Could you check a few things on this model? Use its own coordinates, in mm. Face numbers are marked on the shaded views. A direction names the side the tool comes from. Give positions to 0.01 mm unless a question says otherwise; leave off trailing zeros. Loops run counter-clockwise (first coordinate to the right, second up) from the corner with the lowest first, then second, coordinate; pieces in that order, holes last. Notation, with made-up numbers: (-27, 47) - (23, 47) arc R23 ccw to (23, 57) - close; hole circle Ø11 at (29.25, 44). An arc over 180 degrees is marked (long way). One line per item, written item: value. Start each with the question number.
Q1. I want a section at A-A (z = -18.5). Please give me the cut outline in (x, y), then the cut area to 3 significant figures.
Q2. I want a section at C-C (y = -44). Please give me the cut outline in (x, z), then the cut area to 3 significant figures.
Q3. I want a section at B-B (x = 0). Please give me the cut outline in (y, z), then the cut area to 3 significant figures.
Q4. For the marked faces 1, 2, 3, 4 and 5, which set-ups out of +Z, -Z, +X, -X, +Y, -Y let a thin tool reach every point of the face, with its end or its side?
Q5. I'm going to push flat-ended pins straight in: P1, Ø12, axis at y = -42.5, z = -20, coming from the -X side; P2, Ø2.5, axis at y = -17.5, z = -33, coming from the +X side; P3, Ø5.5, axis at x = 6.5, y = -12.5, coming from the -Z side; P4, Ø10, axis at y = -33, z = -12.5, coming from the +X side. Where does each tip first touch, or does it pass through?
Q6. If I drill on line 1 (Y direction, x = 0, z = -27); line 2 (X direction, y = -37.5, z = -8.5); line 3 (Z direction, x = -29.5, y = -33.5), over which ranges is the centre line in solid material (lowest first)? Write a range as from..to.
Q7. I want a section at D-D (x = 16.5). Please give me the cut outline in (y, z).
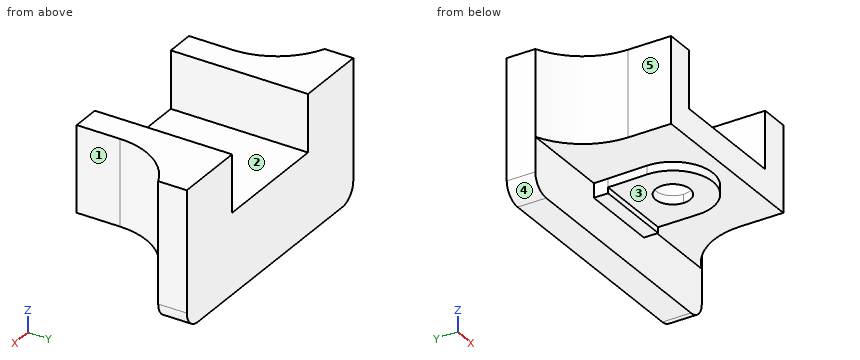
```python
from build123d import *

# Parameters (mm, degrees)
F1_DEPTH    = 48
F2_DEPTH    = 10
F3_R        = 6
F4_DEPTH    = 3
F5_DEPTH    = 5
F6_T1_DEPTH = 30
F7_D        = 12


# Not quite as in the source:
# - a fillet or chamfer that OpenCascade refuses, or shapes differently, is made with other operations: its cross-section is extruded or revolved along the edge and cut away or added


with BuildPart() as f1:
    # F0 (on Front) → F1 (new body)
    with BuildSketch(Plane.XZ):
        Polygon((-21, 0), (-31, 0), (-31, -30), (31, -30), (31, 0), (21, 0), (21, -20), (-21, -20), align=None)
    extrude(amount=F1_DEPTH)

    # F0 (on Front) → F2 (join)
    with BuildSketch(Plane.XZ):
        with BuildLine():
            Line((-31, 0), (-46, 0))
            Line((-46, 0), (-46, -42))
            ThreePointArc((-46, -42), (-44.2426406871, -46.2426406871), (-40, -48))
            Line((-40, -48), (40, -48))
            ThreePointArc((40, -48), (44.2426406871, -46.2426406871), (46, -42))
            Line((46, -42), (46, 0))
            Line((46, 0), (31, 0))
            Line((31, 0), (31, -30))
            Line((31, -30), (-31, -30))
            Line((-31, -30), (-31, 0))
        make_face()
        Polygon((-21, 0), (-31, 0), (-31, -30), (31, -30), (31, 0), (21, 0), (21, -20), (-21, -20), align=None)
    extrude(amount=F2_DEPTH)

    # F3 (on face) → F4 (join)
    with BuildSketch(Plane(origin=(0, 0, -30), x_dir=(1, 0, 0), z_dir=(0, 0, -1))):
        with BuildLine():
            Line((13.9955899146, 15), (13.9955899146, 28.6486270591))
            ThreePointArc((13.9955899146, 28.6486270591), (0.0417417441, 42.9999377722), (-13.9974363474, 28.7320901258))
            Line((-13.9974363474, 28.7320901258), (-13.7346051799, 15))
            Line((-13.7346051799, 15), (13.9955899146, 15))
        make_face()
        with Locations((0, 29)):
            Circle(F3_R, mode=Mode.SUBTRACT)
    extrude(amount=F4_DEPTH)

    # F3 (on face) → F5 (join)
    with BuildSketch(Plane(origin=(0, 0, -30), x_dir=(1, 0, 0), z_dir=(0, 0, -1))):
        Polygon((13.9955899146, 10), (13.9955899146, 15), (-13.7346051799, 15), (-13.6389055576, 10), align=None)
    extrude(amount=F5_DEPTH)

    # F6: fillet of radius 25 on 2 edges, made by hand

    # F6_s2 → F6_t1 (join)
    with BuildSketch(Plane.XY.offset(-30)):
        with BuildLine():
            ThreePointArc((31, -32.9128784748), (35.0834993366, -19.2198145372), (46, -10))
            Line((46, -10), (31, -10))
            Line((31, -10), (31, -32.9128784748))
        make_face()
        with BuildLine():
            ThreePointArc((-46, -10), (-35.0834993366, -19.2198145372), (-31, -32.9128784748))
            Line((-31, -32.9128784748), (-31, -10))
            Line((-31, -10), (-46, -10))
        make_face()
    extrude(amount=F6_T1_DEPTH)

    # F7 (through all)
    with Locations(Plane(origin=(0, 0, -30), x_dir=(1, 0, 0), z_dir=(0, 0, -1))):
        with Locations((0, 29)):
            Hole(F7_D / 2)


solid = f1.part
```
Worked answers:
1. outline: (-46, -10) arc R25 cw to (-31, -32.91) - (-31, -48) - (-21, -48) - (-21, 0) - (-46, 0) - close; (21, -48) - (31, -48) - (31, -32.91) arc R25 cw to (46, -10) - (46, 0) - (21, 0) - close
1. area: 1,450 mm²
2. outline: (-31, -30) - (31, -30) - (31, 0) - (21, 0) - (21, -20) - (-21, -20) - (-21, 0) - (-31, 0) - close
2. area: 1,020 mm²
3. outline: (-48, -30) - (-43, -30) - (-43, -33) - (-35, -33) - (-35, -20) - (-48, -20) - close; (-23, -33) - (-15, -33) - (-15, -35) - (-10, -35) - (-10, -48) - (0, -48) - (0, -20) - (-23, -20) - close
3. area: 613 mm²
4. face 1: +Z, -Z, +X, -Y
4. face 2: +Z, +Y, -Y
4. face 3: -Z, +X, -X, -Y
4. face 4: -Z, -X, +Y, -Y
4. face 5: +Z, -Z, -X, -Y
5. P1: stops at x = -31
5. P2: stops at x = 14
5. P3: stops at z = -48
5. P4: stops at x = 31.49
6. line 1: y = -48..-35, -23..0
6. line 2: x = -31..-21, 21..31
6. line 3: z = -30..0
7. outline: (-48, -30) - (-10, -30) - (-10, -48) - (0, -48) - (0, -20) - (-48, -20) - close
